```python
from build123d import *

# Parameters (mm, degrees)
SKETCH1_R           = 7.5
BOSS_EXTRUDE1_DEPTH = 5


with BuildPart() as part:
    # Sketch1 → Boss-Extrude1 (new body)
    with BuildSketch(Plane.YZ):
        with BuildLine():
            Line((-230, 15), (230, 15))
            ThreePointArc((230, 15), (245, 0), (230, -15))
            Line((230, -15), (-230, -15))
            ThreePointArc((-230, -15), (-245, 0), (-230, 15))
        make_face()
        with Locations(Location((-230, 0, 0), (0, 0, 270))):
            Circle(SKETCH1_R, mode=Mode.SUBTRACT)
        with Locations(Location((0, 0, 0), (0, 0, 270))):
            Circle(SKETCH1_R, mode=Mode.SUBTRACT)
        with Locations(Location((230, 0, 0), (0, 0, 270))):
            Circle(SKETCH1_R, mode=Mode.SUBTRACT)
    extrude(amount=-BOSS_EXTRUDE1_DEPTH)


solid = part.part
```
For this review, take the finished solid that the model builds, in its own axes (mm). Coordinates: 2 decimals unless noted, no trailing zeros. Order: outer loops, then holes, each group sorted by start corner. A loop starts at its lowest first (then second) coordinate and runs counter-clockwise, first axis right, second up. Notation, with made-up numbers: (26, 58) -> (74, 58) arc R26 cw to (74, 84) -> close; hole circle Ø2 at (16.5, -20). An arc over 180 degrees is marked (long way). Answer as CSV lines item,"result".
Q1. We need section B-B (x = -0.9). State the section outline as (y, z) points.
Model answer:
outline,"(-230, -15) -> (230, -15) arc R15 ccw to (230, 15) -> (-230, 15) arc R15 ccw to start; hole circle Ø15 at (-230, 0); hole circle Ø15 at (0, 0); hole circle Ø15 at (230, 0)"
Q2. We need section A-A (y = 0). State the section outline as (x, z) points, plus the area to 3 significant figures.
Model answer:
outline,"(-5, -15) -> (0, -15) -> (0, -7.5) -> (-5, -7.5) -> close; (-5, 7.5) -> (0, 7.5) -> (0, 15) -> (-5, 15) -> close"
area,"75.0 mm2"
Q3. Clearance check with a flat-ended pin moving along its axis: pin 1 Ø12 at (y, z) = (0, 0) entering from -X. State where the tip first meets the part, or that it passes through.
Model answer:
pin 1,"passes through"
Q4. Wall thickness on line 1 along Y through (x, z) = (-2, 0); line 2 along Y through (x, z) = (-0.95, -2.5); line 3 along Y through (x, z) = (-3.6, -10.5): over which ranges is each line inside the solid? List them lowest first. Write a range as [from, to].
Model answer:
line 1,"y = [-245, -237.5], [-222.5, -7.5], [7.5, 222.5], [237.5, 245]"
line 2,"y = [-244.79, -237.07], [-222.93, -7.07], [7.07, 222.93], [237.07, 244.79]"
line 3,"y = [-240.71, 240.71]"
Q5. Draft analysis for pull direction Y (two halves, no side actions). For faces 1 (the face through (-2.465, 237.436, 0.976)), 2 (the face through (0, 3.4, 6.9)), 3 (the face through (-2.465, -222.564, 0.976)), 4 (the face through (-2, -245, 0)), state which applies: released by +Y, released by -Y, zero draft, split by the parting line, or undercut.
Model answer:
face 1,"undercut"
face 2,"zero draft"
face 3,"undercut"
face 4,"released by -Y"
